Autodesk Inventor part; units mm, degrees
ref_plane "YZ Plane" through (0, 0, 0) normal (1, 0, 0) x (0, 1, 0)
ref_plane "XZ Plane" through (0, 0, 0) normal (0, 1, 0) x (-1, 0, 0)
ref_plane "XY Plane" through (0, 0, 0) normal (0, 0, 1) x (1, 0, 0)
sketch "스케치1" plane through (0, 0, 0) normal (0, 0, 1) x (1, 0, 0)
  point P0 (0, 0)
sketch "스케치2" plane through (0, 0, 0) normal (0, 0, 1) x (1, 0, 0)
  line L0 (0, 0) -> (198, 0)
  line L1 (198, 0) -> (198, -30)
  line L2 (198, -30) -> (0, -30)
  line L3 (0, -30) -> (0, 0)
  line L4 (2, -2) -> (28, -2)
  line L5 (28, -2) -> (28, -28)
  line L6 (28, -28) -> (2, -28)
  line L7 (2, -28) -> (2, -2)
  line L8 (56, -2) -> (56, -28)
  line L9 (30, -2) -> (56, -2)
  line L10 (30, -28) -> (30, -2)
  line L11 (56, -28) -> (30, -28)
  line L12 (84, -2) -> (84, -28)
  line L13 (58, -2) -> (84, -2)
  line L14 (58, -28) -> (58, -2)
  line L15 (84, -28) -> (58, -28)
  line L16 (112, -2) -> (112, -28)
  line L17 (86, -2) -> (112, -2)
  line L18 (86, -28) -> (86, -2)
  line L19 (112, -28) -> (86, -28)
  line L20 (140, -2) -> (140, -28)
  line L21 (114, -2) -> (140, -2)
  line L22 (114, -28) -> (114, -2)
  line L23 (140, -28) -> (114, -28)
  line L24 (168, -2) -> (168, -28)
  line L25 (142, -2) -> (168, -2)
  line L26 (142, -28) -> (142, -2)
  line L27 (168, -28) -> (142, -28)
  line L28 (196, -2) -> (196, -28)
  line L29 (170, -2) -> (196, -2)
  line L30 (170, -28) -> (170, -2)
  line L31 (196, -28) -> (170, -28)
  dimension "d0" = 198
  dimension "d1" = 30
  dimension "d2" = 2
  dimension "d3" = 2
  dimension "d4" = 26
  dimension "d5" = 26
  dimension "d8" = 28
extrude "돌출1" add sketch "스케치2" along normal blind 4
sketch "스케치3" plane through (0, 0, 4) normal (0, 0, 1) x (1, 0, 0)
  line L0 (0, -30) -> (198, -30)
  line L1 (198, -30) -> (198, 0)
  line L2 (198, 0) -> (0, 0)
  line L3 (0, 0) -> (0, -30)
  line L4 (196, -2) -> (196, -28)
  line L5 (196, -28) -> (170, -28)
  line L6 (170, -28) -> (170, -2)
  line L7 (170, -2) -> (196, -2)
  line L8 (168, -2) -> (168, -28)
  line L9 (168, -28) -> (142, -28)
  line L10 (142, -28) -> (142, -2)
  line L11 (142, -2) -> (168, -2)
  line L12 (140, -2) -> (140, -28)
  line L13 (140, -28) -> (114, -28)
  line L14 (114, -28) -> (114, -2)
  line L15 (114, -2) -> (140, -2)
  line L16 (112, -2) -> (112, -28)
  line L17 (112, -28) -> (86, -28)
  line L18 (86, -28) -> (86, -2)
  line L19 (86, -2) -> (112, -2)
  line L20 (84, -2) -> (84, -28)
  line L21 (84, -28) -> (58, -28)
  line L22 (58, -28) -> (58, -2)
  line L23 (58, -2) -> (84, -2)
  line L24 (56, -2) -> (56, -28)
  line L25 (56, -28) -> (30, -28)
  line L26 (30, -28) -> (30, -2)
  line L27 (30, -2) -> (56, -2)
  line L28 (2, -2) -> (28, -2)
  line L29 (28, -2) -> (28, -28)
  line L30 (28, -28) -> (2, -28)
  line L31 (2, -28) -> (2, -2)
extrude "돌출2" add sketch "스케치3" along normal blind 1 contours L3 L2 L1 L0 | L4 L5 L6 L7 | L8 L9 L10 L11 | L12 L13 L14 L15 | L16 L17 L18 L19 | L20 L21 L22 L23 | L24 L25 L26 L27 | L28 L29 L30 L31
fillet "모깎기1" radius 2 4 edges at (198, 0, 2.5) (198, -30, 2.5) (0, -30, 2.5) (0, 0, 2.5)
properties part number "h_pocket"
The model under review builds one solid part; all positions refer to its coordinate system, in mm. Give positions to 0.01 mm unless a question says otherwise; leave off trailing zeros. Loops run counter-clockwise (first coordinate to the right, second up) from the corner with the lowest first, then second, coordinate; pieces in that order, holes last. Notation, with made-up numbers: (83.5, 27) -> (132.5, 27) arc R23 cw to (132.5, 43) -> close; hole circle Ø3 at (14, 70). An arc over 180 degrees is marked (long way). Put each result on its own line as item: value. Start each with the question number.
1. Wall thickness on probe 1 along Y at (x, z) = (98, 0.5); probe 2 along Z at (x, y) = (180, -9): over which ranges is each line inside the solid? List them lowest first.
2. Clearance check with flat-ended pins moving along their axes: P1, Ø2, axis at x = 97.5, z = 2, coming from the +Y side; P2, Ø3, axis at x = 134, y = -24, coming from the -Z side. State where each tip first meets the part, or that it passes through.
3. Mouldability with a two-part tool opening along Y and no side actions: class faces 1 (the face through (98, 0, 2)), 2 (the face through (114, -15, 2)), 3 (the face through (100, -30, 2)) as released by +Y, released by -Y, zero draft, split by the parting line, or undercut.
4. We need section B-B on x = 75.5. State the section outline as (y, z) points.
5. We need section C-C on z = 1.1. State how many separate pieces and enclosed holes the cut face has, then the cut area to 3 significant figures.
Determined:
1. probe 1: -30 to -28, -2 to 0
1. probe 2: 4 to 5
2. P1: y = 0
2. P2: z = 4
3. face 1: released by +Y
3. face 2: undercut
3. face 3: released by -Y
4. outline: (-30, 0) -> (-28, 0) -> (-28, 4) -> (-2, 4) -> (-2, 0) -> (0, 0) -> (0, 5) -> (-30, 5) -> close
5. separate pieces: 1
5. enclosed holes: 7
5. area: 1,200 mm^2
